from build123d import *

# Parameters (mm, degrees)
SKETCH_1_R      = 2.5
EXTRUDE_1_DEPTH = 0.2
SKETCH_2_R      = 1
EXTRUDE_2_DEPTH = 6
SKETCH_3_R      = 2
EXTRUDE_3_DEPTH = 1.2
EXTRUDE_3_TAPER = 30


with BuildPart() as part:
    # 스케치1 → 보스-돌출1 (new body)
    with BuildSketch(Plane(origin=(0, 0, 0), x_dir=(1, 0, 0), z_dir=(0, 1, 0))):
        with Locations(Location((0, 0, 0), (0, 0, 270))):
            Circle(SKETCH_1_R)
    extrude(amount=EXTRUDE_1_DEPTH)

    # 스케치2 → 보스-돌출2 (add)
    with BuildSketch(Plane.XZ):
        with Locations(Location((0, 0, 0), (0, 0, 270))):
            Circle(SKETCH_2_R)
    extrude(amount=EXTRUDE_2_DEPTH)

    # 스케치3 → 보스-돌출3 (add)
    with BuildSketch(Plane(origin=(0, 0.2, 0), x_dir=(1, 0, 0), z_dir=(0, 1, 0))):
        Circle(SKETCH_3_R)
    extrude(amount=EXTRUDE_3_DEPTH, taper=EXTRUDE_3_TAPER)


solid = part.part
Verification items for the finished model (mm, model axes). A direction names the side the tool comes from. Round coordinates to 2 decimals unless told otherwise and drop trailing zeros. Order: outer loops, then holes, each group sorted by start corner. A loop starts at its lowest first (then second) coordinate and runs counter-clockwise, first axis right, second up. Notation, with made-up numbers: (-1.5, 3.25) -> (34.5, 3.25) arc R24 cw to (34.5, 29.25) -> close; hole circle Ø3 at (-31.75, -27). An arc over 180 degrees is marked (long way). Put each result on its own line as item: value.
1) Section check C-C (x = 2.15). Record the cut outline in (y, z), then the cut area to 3 significant figures.
Final values:
outline: (0, -1.28) -> (0.2, -1.28) -> (0.2, 1.28) -> (0, 1.28) -> close
area: 0.510 mm^2
2) Section check A-A (x = 0). Record the cut outline in (y, z), then the cut area to 3 significant figures.
Final values:
outline: (-6, -1) -> (0, -1) -> (0, -2.5) -> (0.2, -2.5) -> (0.2, -2) -> (1.4, -1.31) -> (1.4, 1.31) -> (0.2, 2) -> (0.2, 2.5) -> (0, 2.5) -> (0, 1) -> (-6, 1) -> close
area: 17.0 mm^2
3) Section check D-D (y = 1). Record the cut outline in (x, z).
Final values:
outline: circle Ø3.08 at (0, 0)
4) Depth check by flat-ended pin: pin 1 (1.5 mm diameter, centred on x = 0.5, y = -5, fed in from +Z). Enter the tip coordinate at first touch or a pass-through.
Final values:
pin 1: stops at z = 1
5) Section check B-B (y = -4.5). Record the cut outline in (x, z), then the cut area to 3 significant figures.
Final values:
outline: circle Ø2 at (0, 0)
area: 3.14 mm^2
6) Set-up check for faces 1 (the flat face through (0, -6, 0)), 2 (the flat face through (-1, 0, 1)), 3 (the flat face through (2, 0.2, -1)): record each of +Z, -Z, +X, -X, +Y, -Y from which the full face is reachable in a straight line by a thin tool's end or side.
Final values:
face 1: +Z, -Z, +X, -X, -Y
face 2: -Y
face 3: +Y
7) Material ranges on line 1 (Y direction, x = 1.7, z = -1.7); line 2 (X direction, y = -1.75, z = 0.05); line 3 (Y direction, x = 0, z = 1.1), recorded low to high.
Final values:
line 1: y = 0 to 0.2
line 2: x = -1 to 1
line 3: y = 0 to 1.4
